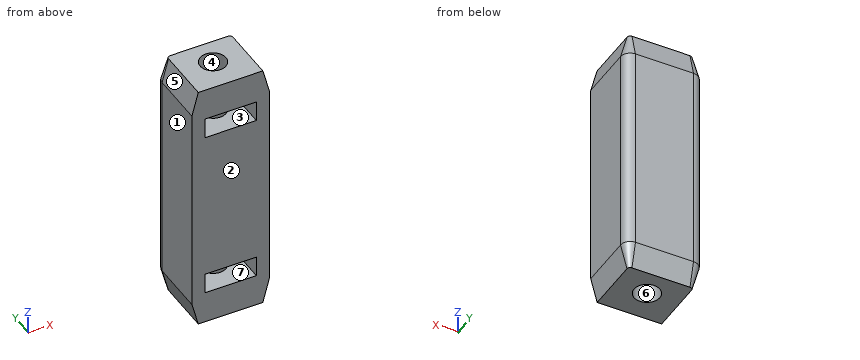
Autodesk Fusion 360 part; units mm, degrees
sketch "Sketch1" plane through (0, 0, 0) normal (0, 0, 1) x (1, 0, 0)
  line L0 (3, -2.5) -> (-3, -2.5)
  line L1 (-3, -2.5) -> (-3, 2.5)
  line L2 (-3, 2.5) -> (3, 2.5)
  line L3 (3, 2.5) -> (3, -2.5)
  line L4 (3, -2.5) -> (-3, 2.5) construction
  line L5 (-3, -2.5) -> (3, 2.5) construction
  dimension "dWidth" = 6
  dimension "d2" = 5
extrude "Extrude1" add sketch "Sketch1" along normal blind 10
sketch "Sketch2" plane through (0, 0, 10) normal (0, 0, 1) x (1, 0, 0)
  line L0 (3, 2.5) -> (-3, 2.5)
  line L1 (-3, 2.5) -> (-3, -2.5)
  line L2 (-3, -2.5) -> (3, -2.5)
  line L3 (3, -2.5) -> (3, 2.5)
  circle A0 centre (0, 0) radius 1
  dimension "d5" = 2
extrude "Extrude2" cut sketch "Sketch2" against normal blind 7 contours A0
ref_plane "WorkPlane1" through (0, 0, 7.5) normal (0, 0, 1) x (1, 0, 0)
sketch "Sketch3" plane through (0, 0, 7.5) normal (0, 0, 1) x (1, 0, 0)
  line L0 (2, -2.16) -> (-2, -2.16) construction
  line L1 (-2, -2.16) -> (-2, 2.16) construction
  line L2 (-2, 2.16) -> (2, 2.16) construction
  line L3 (2, 2.16) -> (2, -2.16) construction
  line L4 (2, -2.16) -> (-2, 2.16) construction
  line L5 (-2, -2.16) -> (2, 2.16) construction
  line L6 (-2, 0) -> (2, 0) construction
  line L7 (2, 1.1258) -> (2, -1.1258)
  line L8 (-2, 1.1258) -> (-2, -1.1258)
  line L9 (0, 2.16) -> (0, -2.16) construction
  line L10 (-2, 1.1258) -> (0, 2.16)
  line L11 (2, 1.1258) -> (0, 2.16)
  line L12 (-2, -1.1258) -> (0, -2.16) construction
  line L13 (0, -2.16) -> (2, -1.1258) construction
  line L14 (-2, -1.1258) -> (-2, -2.5)
  line L15 (-2, -2.5) -> (2, -2.5)
  line L16 (2, -2.5) -> (2, -1.1258)
  line L17 (3, -2.5) -> (-3, -2.5)
  dimension "d9" = 4
  dimension "d10" = 4.32
extrude "Extrude3" cut sketch "Sketch3" against normal blind 1.6
fillet "Fillet1" radius 0.75 2 edges at (-3, 2.5, 5) (3, 2.5, 5)
chamfer "Chamfer2" distance 0.5 angle 75 2 edges at (3, -0.375, 10) (-3, -0.375, 10) measured on face at (-2.3296, -0.2997, 10) measured on face at (-2.3296, -0.2997, 10)
mirror "Mirror2" about plane through (0, 0, 0) normal (0, 0, 1) of bodies 1 merged
properties part number "Configuration 2"
Geometry: final body of the model. Coordinates: model frame, mm. Face numbers are marked on the shaded views. A direction names the side the tool comes from. Round coordinates to 2 decimals unless told otherwise and drop trailing zeros. Order: outer loops, then holes, each group sorted by start corner. A loop starts at its lowest first (then second) coordinate and runs counter-clockwise, first axis right, second up. Notation, with made-up numbers: (13.5, 20) -> (68.5, 20) arc R19 ccw to (68.5, 54) -> close; hole circle Ø3 at (-1, 61.5). An arc over 180 degrees is marked (long way). Use one line per item in the form item = value.
(1) Access query for the marked faces 5, 6 and 7. Directions: +Z, -Z, +X, -X, +Y, -Y. A direction counts if a zero-diameter tool reaches every point of the face in a straight line with its end or side. Return the directions, or none.
Results list:
face_5 = +Z, -X, +Y, -Y
face_6 = -Z
face_7 = -Y
(2) Draft query along X for the marked faces 1, 2, 3 and 4. Return one class per face: pulls with the +X half, pulls with the -X half, needs draft (parallel to the pull), parting line crosses it, or undercut.
Results list:
face_1 = pulls with the -X half
face_2 = needs draft
face_3 = undercut
face_4 = undercut
(3) Ray query, probe 1 along Z at (x, y) = (-1.5, -0.45); probe 2 along Y at (x, z) = (0, -4.95); probe 3 along X at (y, z) = (-0.1, 5.5). Return the intervals inside material, ascending. Write a range as [from, to].
Results list:
probe_1 = [-10, -7.5], [-5.9, 5.9], [7.5, 10]
probe_2 = [-2.5, -1], [1, 2.5]
probe_3 = [-3, -0.99], [0.99, 3]
(4) Section D-D on z = 8.75. Return loops of the section in (x, y).
Results list:
outline = (-2.83, -2.5) -> (2.83, -2.5) -> (2.83, 1.75) arc R0.58 ccw to (2.25, 2.33) -> (-2.25, 2.33) arc R0.58 ccw to (-2.83, 1.75) -> close; hole circle Ø2 at (0, 0)
(5) Section A-A on z = -3.75. Return loops of the section in (x, y).
Results list:
outline = (-3, -2.5) -> (3, -2.5) -> (3, 1.75) arc R0.75 ccw to (2.25, 2.5) -> (-2.25, 2.5) arc R0.75 ccw to (-3, 1.75) -> close; hole circle Ø2 at (0, 0)
(6) First-contact query: pin 1 Ø1.6 at (x, y) = (0.5, 0) entering from +Z; pin 2 Ø1 at (x, y) = (0, 0) entering from -Z; pin 3 Ø1.2 at (x, y) = (0, 0) entering from +Z. Flat tips, straight axial feed; report the tip coordinate or a pass-through.
Results list:
pin_1 = 10
pin_2 = -3
pin_3 = 3
(7) Section B-B on x = -0.25. Count the separate pieces of the cut face and the enclosed holes in it, and give its area (3 significant figures).
Results list:
separate_pieces = 3
enclosed_holes = 0
area = 63.7 mm^2
